```python
from build123d import *

# Parameters (mm, degrees)
SKETCH1_R                        = 25.9
BOSS_EXTRUDE1_DEPTH              = 76.2
SKETCH2_R                        = 15.9
CUT_EXTRUDE1_DEPTH               = 75
F_10_5_10_5_DIAMETER_HOLE1_D     = 10.5
F_10_5_10_5_DIAMETER_HOLE1_DEPTH = 20
F_10_5_10_5_DIAMETER_HOLE1_TIP   = 3.15451825
F_12_8_12_8_DIAMETER_HOLE1_D     = 12.8
F_12_8_12_8_DIAMETER_HOLE1_DEPTH = 300
F_12_8_12_8_DIAMETER_HOLE1_TIP   = 3.845507962


with BuildPart() as part:
    # Sketch1 → Boss-Extrude1 (new body)
    with BuildSketch(Plane.XY):
        Circle(SKETCH1_R)
    extrude(amount=BOSS_EXTRUDE1_DEPTH)

    # Sketch2 → Cut-Extrude1 (cut)
    with BuildSketch(Plane.XY.offset(76.2)):
        Circle(SKETCH2_R)
    extrude(amount=-CUT_EXTRUDE1_DEPTH, mode=Mode.SUBTRACT)

    # Ø10.5 (10.5) Diameter Hole1
    with Locations(Plane(origin=(5.482930922, 25.312990114, 25), x_dir=(0.977335526, -0.211696175, 0), z_dir=(0.211696175, 0.977335526, 0))):
        with Locations((0, 0)):
            Hole(F_10_5_10_5_DIAMETER_HOLE1_D / 2, depth=F_10_5_10_5_DIAMETER_HOLE1_DEPTH)
            with Locations((0, 0, -(F_10_5_10_5_DIAMETER_HOLE1_DEPTH + F_10_5_10_5_DIAMETER_HOLE1_TIP / 2))):  # 118° drill point
                Cone(0, F_10_5_10_5_DIAMETER_HOLE1_D / 2, F_10_5_10_5_DIAMETER_HOLE1_TIP, mode=Mode.SUBTRACT)

    # Ø12.8 (12.8) Diameter Hole1
    with Locations(Plane(origin=(5.555887044, 25.297073879, 60), x_dir=(0.976721125, -0.214513041, 0), z_dir=(0.214513041, 0.976721125, 0))):
        with Locations((0, 0)):
            Hole(F_12_8_12_8_DIAMETER_HOLE1_D / 2, depth=F_12_8_12_8_DIAMETER_HOLE1_DEPTH)
            with Locations((0, 0, -(F_12_8_12_8_DIAMETER_HOLE1_DEPTH + F_12_8_12_8_DIAMETER_HOLE1_TIP / 2))):  # 118° drill point
                Cone(0, F_12_8_12_8_DIAMETER_HOLE1_D / 2, F_12_8_12_8_DIAMETER_HOLE1_TIP, mode=Mode.SUBTRACT)


solid = part.part
```
The model under review builds one solid part; all positions refer to its coordinate system, in mm. A direction names the side the tool comes from. Give positions to 0.01 mm unless a question says otherwise; leave off trailing zeros. Write each loop counter-clockwise with the first axis right and the second up, starting at its lowest first coordinate (ties: lowest second). Pieces come first, ordered by that corner, then holes. Notation, with made-up numbers: M 79.5,-39.75 L 88.5,-39.75 A9 cw 88.5,-24.75 Z; hole C 78.25,-29 d4. An arc over 180 degrees is marked long. Answer in a Markdown table with one row per item.
Item 1: Add section A-A on z = 64. Give the boundary of the cut face in (x, y), plus the area to 3 significant figures.
Check sheet entries:
| item | result |
|---|---|
| outline | M -10.33,-23.75 L -8.12,-13.67 A15.9 cw -1.64,15.82 L 0.57,25.89 A25.9 ccw Z; M -0.57,-25.89 A25.9 ccw 10.33,23.75 L 8.12,13.67 A15.9 cw 1.64,-15.82 Z |
| area | 1,110 mm2 |
Item 2: Add section C-C on z = 44.5. Give the boundary of the cut face in (x, y).
Check sheet entries:
| item | result |
|---|---|
| outline | C 0,0 d51.8; hole C 0,0 d31.8 |
Item 3: Draft analysis for pull direction X (two halves, no side actions). For faces 3 (the face through (0, 0, 1.2)), 4 (the face through (0, 0, 0)), 5 (the face through (-3.37, 25.68, 37.57)), state which applies: +X half, -X half, draft (parallel to the pull), parting line (faces both ways), or undercut.
Check sheet entries:
| item | result |
|---|---|
| face 3 | undercut |
| face 4 | draft |
| face 5 | parting line |
Item 4: Add section B-B on y = 0. Give the boundary of the cut face in (x, z), plus the area to 3 significant figures.
Check sheet entries:
| item | result |
|---|---|
| outline | M -25.9,0 L 25.9,0 L 25.9,76.2 L 15.9,76.2 L 15.9,1.2 L -15.9,1.2 L -15.9,76.2 L -25.9,76.2 Z |
| area | 1,560 mm2 |
Item 5: For P1, Ø1.5, axis at x = -8.5, z = 32, coming from the -Y side; P2, Ø4, axis at x = -7.5, z = 59.5, coming from the +Y side; P3, Ø4, axis at y = 7, z = 66.5, coming from the +X side, all flat-tipped, find the tip position at first contact; note any pin that passes through.
Check sheet entries:
| item | result |
|---|---|
| P1 | y = -24.71 |
| P2 | y = 25.31 |
| P3 | x = 25.41 |
Item 6: For line 1 along Z through (x, y) = (-7.5, 12); line 2 along Y through (x, z) = (0.5, 5); line 3 along Y through (x, z) = (-6, 13.5), list the stretches that pass through material, from the lowest coordinate up.
Check sheet entries:
| item | result |
|---|---|
| line 1 | 0 to 1.2 |
| line 2 | -25.9 to -15.89, 15.89 to 25.9 |
| line 3 | -25.2 to -14.72, 14.72 to 25.2 |
Item 7: Add section D-D on x = 5. State how many separate pieces and enclosed holes the cut face has, plus the area to 3 significant figures.
Check sheet entries:
| item | result |
|---|---|
| separate pieces | 3 |
| enclosed holes | 0 |
| area | 1,370 mm2 |
Item 8: Tool access review of faces 1 (the face through (-2.07, 15.765, 39.225)), 2 (the face through (-12, -11, 76.2)): name each direction out of +Z, -Z, +X, -X, +Y, -Y from which nothing blocks a thin tool from reaching the whole face with its end or side.
Check sheet entries:
| item | result |
|---|---|
| face 1 | +Z |
| face 2 | +Z, +X, -X, +Y, -Y |
